Design review of the part built by this model. Coordinates are the model's own, in mm. Give positions to 0.01 mm unless a question says otherwise; leave off trailing zeros. Loops run counter-clockwise (first coordinate to the right, second up) from the corner with the lowest first, then second, coordinate; pieces in that order, holes last. Notation, with made-up numbers: (18.25, 52.25) - (58.25, 52.25) arc R9 cw to (58.25, 62.25) - close; hole circle Ø11 at (62, -37). An arc over 180 degrees is marked (long way). Write each question's results on one line, items separated by ' | '.
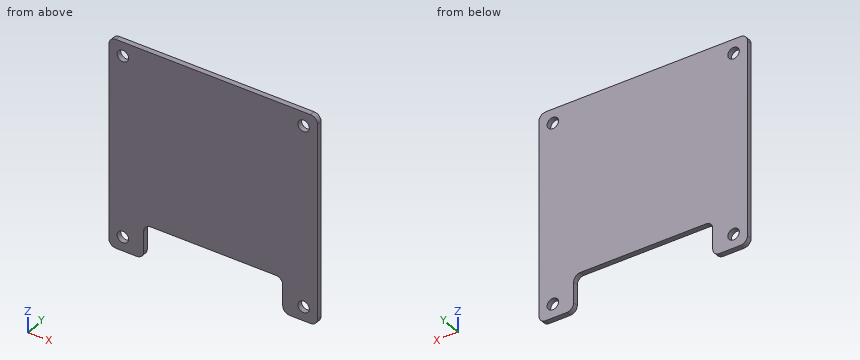
```python
from build123d import *

# Parameters (mm, degrees)
SKETCH_1_R      = 1.65
EXTRUDE_1_DEPTH = 1.5
FILLET_1_R      = 2
FILLET_2_R      = 2


with BuildPart() as part:
    # Эскиз1 → Бобышка-Вытянуть1 (new body)
    with BuildSketch(Plane(origin=(0, 0, 0), x_dir=(1, 0, 0), z_dir=(0, 1, 0))):
        with BuildLine():
            Line((20, 30), (30, 30))
            Line((30, 30), (30, -30))
            Line((30, -30), (-30, -30))
            Line((-30, -30), (-30, 30))
            Line((-30, 30), (-20, 30))
            Line((-20, 30), (-20, 22))
            ThreePointArc((-20, 22), (-19.414213562, 20.585786438), (-18, 20))
            Line((-18, 20), (18, 20))
            ThreePointArc((18, 20), (19.414213562, 20.585786438), (20, 22))
            Line((20, 22), (20, 30))
        make_face()
        with Locations(Location((-26, 26, 0), (0, 0, 270))):
            Circle(SKETCH_1_R, mode=Mode.SUBTRACT)
        with Locations(Location((26, 26, 0), (0, 0, 270))):
            Circle(SKETCH_1_R, mode=Mode.SUBTRACT)
        with Locations(Location((-26, -26, 0), (0, 0, 270))):
            Circle(SKETCH_1_R, mode=Mode.SUBTRACT)
        with Locations(Location((26, -26, 0), (0, 0, 270))):
            Circle(SKETCH_1_R, mode=Mode.SUBTRACT)
    extrude(amount=EXTRUDE_1_DEPTH)

    # Скругление1
    fillet_1_edges = [part.edges().sort_by_distance(p)[0] for p in [
        (-30, 0.75, 30),
    ]]
    fillet(fillet_1_edges, radius=FILLET_1_R)

    # Скругление2
    fillet_2_edges = [part.edges().sort_by_distance(p)[0] for p in [
        (-30, 0.75, -30),
        (-20, 0.75, -30),
        (20, 0.75, -30),
        (30, 0.75, -30),
        (30, 0.75, 30),
    ]]
    fillet(fillet_2_edges, radius=FILLET_2_R)


solid = part.part
```
Item 1: We need section C-C on z = 26. Give the boundary of the cut face in (x, y), then the cut area to 3 significant figures.
Output values:
outline: (-30, 0) - (-27.65, 0) - (-27.65, 1.5) - (-30, 1.5) - close; (-24.35, 0) - (24.35, 0) - (24.35, 1.5) - (-24.35, 1.5) - close; (27.65, 0) - (30, 0) - (30, 1.5) - (27.65, 1.5) - close | area: 80.1 mm²
Item 2: We need section A-A on x = 26. Give the boundary of the cut face in (y, z).
Output values:
outline: (0, -30) - (1.5, -30) - (1.5, -27.65) - (0, -27.65) - close; (0, -24.35) - (1.5, -24.35) - (1.5, 24.35) - (0, 24.35) - close; (0, 27.65) - (1.5, 27.65) - (1.5, 30) - (0, 30) - close
Item 3: Wall thickness on probe 1 along X at (y, z) = (1.15, -26); probe 2 along X at (y, z) = (0.9, 26); probe 3 along Z at (x, y) = (-27, 0.3): over which ranges is each line inside the solid? List them lowest first.
Output values:
probe 1: x = -30 to -27.65, -24.35 to -20, 20 to 24.35, 27.65 to 30 | probe 2: x = -30 to -27.65, -24.35 to 24.35, 27.65 to 30 | probe 3: z = -30 to -27.31, -24.69 to 24.69, 27.31 to 30
Item 4: We need section B-B on y = 0.6. Give the boundary of the cut face in (x, z), then the cut area to 3 significant figures.
Output values:
outline: (-30, -28) arc R2 ccw to (-28, -30) - (-22, -30) arc R2 ccw to (-20, -28) - (-20, -22) arc R2 cw to (-18, -20) - (18, -20) arc R2 cw to (20, -22) - (20, -28) arc R2 ccw to (22, -30) - (28, -30) arc R2 ccw to (30, -28) - (30, 28) arc R2 ccw to (28, 30) - (-28, 30) arc R2 ccw to (-30, 28) - close; hole circle Ø3.3 at (-26, -26); hole circle Ø3.3 at (-26, 26); hole circle Ø3.3 at (26, -26); hole circle Ø3.3 at (26, 26) | area: 3,160 mm²
Item 5: Clearance check with a flat-ended pin moving along its axis: P1, Ø0.8, axis at x = 1, y = 1, coming from the -Z side. State where the tip first meets the part, or that it passes through.
Output values:
P1: stops at z = -20
Item 6: We need section D-D on x = -5. Give the boundary of the cut face in (y, z).
Output values:
outline: (0, -20) - (1.5, -20) - (1.5, 30) - (0, 30) - close
